from build123d import *

# Parameters (mm, degrees)
GUIDE_START        = 3.429
GUIDE_VANES_DEPTH  = 17.78
CIRPATTERN4_COUNT  = 10
SKETCH6_R          = 1.7526
CUT_EXTRUDE1_DEPTH = 13.97
CIRPATTERN5_COUNT  = 4
SKETCH9_R          = 4.7625
CUT_EXTRUDE2_DEPTH = 7.62


with BuildPart() as part:
    # Sketch3 → Body (revolve)
    with BuildSketch(Plane.XY):
        Polygon((-69.85, 16.0734375), (-39.624, 16.0734375), (-39.624, 10.4854375), (0, 10.4854375), (0, 3.3734375), (-69.85, 3.3734375), align=None)
    revolve(axis=Axis((0, 0, 0), (0, 1, 0)))

    # Sketch4 → Guide Vanes (add)
    with BuildSketch(Plane(origin=(0, 0, 0), x_dir=(1, 0, 0), z_dir=(0, 1, 0)).offset(GUIDE_START)):
        with BuildLine():
            Line((1.553349961, 52.076946284), (26.95018459, 71.275013508))
            ThreePointArc((26.95018459, 71.275013508), (36.029244063, 67.144125374), (44.490941148, 61.862720242))
            Line((44.490941148, 61.862720242), (1.553349961, 52.076946284))
        make_face()
    guide_vanes = extrude(amount=GUIDE_VANES_DEPTH)

    # CirPattern4: Guide Vanes ×10 about axis
    cirpattern4_axis = Axis((0, 0, 0), (0, 1, 0))
    for i in range(1, CIRPATTERN4_COUNT):
        add(guide_vanes.rotate(cirpattern4_axis, i * 360 / CIRPATTERN4_COUNT))

    # Sketch6 → Cut-Extrude1 (cut)
    with BuildSketch(Plane(origin=(0, 0, 0), x_dir=(1, 0, 0), z_dir=(0, 1, 0))):
        with Locations((0, 17.78)):
            Circle(SKETCH6_R)
    cut_extrude1 = extrude(amount=CUT_EXTRUDE1_DEPTH, mode=Mode.SUBTRACT)

    # CirPattern5: Cut-Extrude1 ×4 about axis
    cirpattern5_axis = Axis((0, 0, 0), (0, 1, 0))
    for i in range(1, CIRPATTERN5_COUNT):
        add(cut_extrude1.rotate(cirpattern5_axis, i * 360 / CIRPATTERN5_COUNT), mode=Mode.SUBTRACT)

    # Sketch9 → Cut-Extrude2 (cut)
    with BuildSketch(Plane(origin=(0, 10.4854375, 0), x_dir=(1, 0, 0), z_dir=(0, 1, 0))):
        Circle(SKETCH9_R)
    extrude(amount=-CUT_EXTRUDE2_DEPTH, mode=Mode.SUBTRACT)


solid = part.part
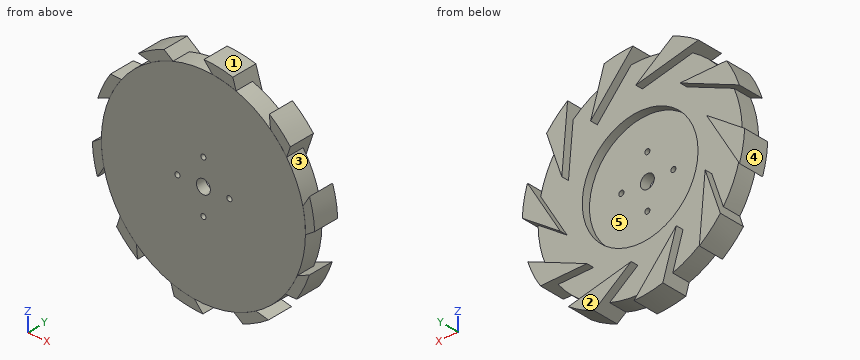
Source: CAD feature listing. Evaluate the final solid. Frame: model axes, mm. Face numbers are marked on the shaded views. A direction names the side the tool comes from. Give positions to 0.01 mm unless a question says otherwise; leave off trailing zeros. Write each loop counter-clockwise with the first axis right and the second up, starting at its lowest first coordinate (ties: lowest second). Pieces come first, ordered by that corner, then holes. Notation, with made-up numbers: M 78.5,62 L 83.5,62 A26 cw 83.5,93 Z; hole C 17.5,6 d10. An arc over 180 degrees is marked long. Return JSON: item names as keys, results as strings. Group by question number.
1) Cut plane D-D, the plane y = 5.5. Give the number of separate pieces and of enclosed holes in the cut face, then the cut area to 3 significant figures.
2) Cut plane A-A, the plane x = -17.78. Output: boundary loops of the cut face in (y, z).
3) Set-up query: the marked faces 4 and 5. Return all of +Z, -Z, +X, -X, +Y, -Y with unobstructed straight access to the full face (end or side cutting, diameter ignored); none if empty.
4) Ray query, L1, parallel to X at y = 11.75, z = -26.5; L2, parallel to X at y = 8.75, z = 0; L3, parallel to Y at x = 45, z = 14. Return the intervals inside material, ascending.
5) Cut plane B-B, the plane z = -7.5. Output: boundary loops of the cut face in (x, y), then the cut area to 3 significant figures.
6) Draft query along X for the marked faces 1, 2 and 3. Return one class per face: released by +X, released by -X, zero draft, split by the parting line, or undercut.
7) First-contact query: pin 1 Ø3.5 at (x, z) = (-28, 68) entering from -Y; pin 2 Ø3 at (x, y) = (-28.5, 11.5) entering from +Z; pin 3 Ø1.5 at (x, y) = (-45.5, 18) entering from +Z. Flat tips, straight axial feed; report the tip coordinate or a pass-through.
8) Cut plane C-C, the plane x = 9.5. Output: boundary loops of the cut face in (y, z).
Data:
{
 "1": {"separate pieces": "1", "enclosed holes": "5", "area": "16,400 mm²"},
 "2": {"outline": "M 3.37,-67.55 L 3.43,-67.55 L 3.43,-74.1 L 21.21,-74.1 L 21.21,-56.28 L 16.07,-56.28 L 16.07,-35.41 L 10.49,-35.41 L 10.49,-1.75 L 3.37,-1.75 Z; M 3.37,1.75 L 10.49,1.75 L 10.49,35.41 L 16.07,35.41 L 16.07,55.78 L 21.21,55.78 L 21.21,64.34 L 16.07,64.34 L 16.07,67.55 L 3.37,67.55 Z"},
 "3": {"face 4": "-Z, -X, +Y, -Y", "face 5": "+Y"},
 "4": {"L1": "x = -64.63 to -29.46, 29.46 to 64.63, 66.27 to 71.44", "L2": "x = -70.95 to -19.53, -16.03 to -4.76, 4.76 to 16.03, 19.53 to 70.95", "L3": "y = 3.37 to 16.07"},
 "5": {"outline": "M -75.83,3.43 L -69.45,3.43 L -69.45,3.37 L 69.45,3.37 L 69.45,16.07 L 60.2,16.07 L 60.2,21.21 L 54.26,21.21 L 54.26,16.07 L 38.91,16.07 L 38.91,10.49 L -38.91,10.49 L -38.91,16.07 L -63.21,16.07 L -63.21,21.21 L -75.83,21.21 Z", "area": "1,510 mm²"},
 "6": {"face 1": "released by +X", "face 2": "zero draft", "face 3": "undercut"},
 "7": {"pin 1": "stops at y = 3.43", "pin 2": "stops at z = 71.26", "pin 3": "stops at z = 41.49"},
 "8": {"outline": "M 3.37,-69.2 L 16.07,-69.2 L 16.07,-58.08 L 21.21,-58.08 L 21.21,-53.89 L 16.07,-53.89 L 16.07,-38.47 L 10.49,-38.47 L 10.49,38.47 L 16.07,38.47 L 16.07,65.75 L 21.21,65.75 L 21.21,75.61 L 3.43,75.61 L 3.43,69.2 L 3.37,69.2 Z"}
}
